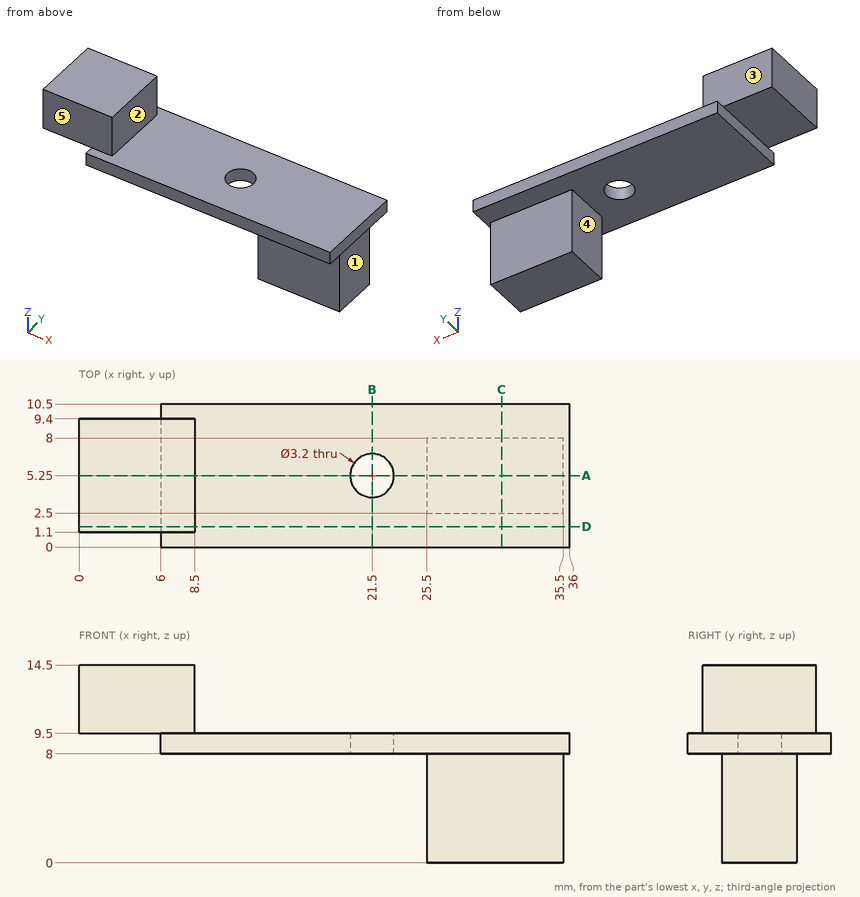
Answer from the drawing. Dimensions are ordinates in mm from the lowest x, y and z of the part. A direction names the side the tool comes from. Round coordinates to 2 decimals unless told otherwise and drop trailing zeros. Write each loop counter-clockwise with the first axis right and the second up, starting at its lowest first coordinate (ties: lowest second). Pieces come first, ordered by that corner, then holes. Notation, with made-up numbers: (5, 69.25) -> (48, 69.25) arc R14 cw to (48, 73.25) -> close; hole circle Ø4 at (-26.5, -3). An arc over 180 degrees is marked (long way). Answer in a Markdown table with one row per item. Add a question column.
1) Find section C-C, the plane x = 31. Determine the outline of the cut face in (y, z), and give its area (4 significant figures).
2) Find section B-B, the plane x = 21.5. Determine the outline of the cut face in (y, z), and give its area (4 significant figures).
3) Consider line 1 (Y direction, x = 21.5, z = 9.15); line 2 (Z direction, x = 3.5, y = 5.5); line 3 (X direction, y = 6.25, z = 10.5). Determine where each line is inside the solid, lowest interval first.
4) Find section A-A, the plane y = 5.25. Determine the outline of the cut face in (x, z), and give its area (3 significant figures).
5) Given P1, Ø5, axis at x = 28, y = 2.5, coming from the +Z side; P2, Ø3.5, axis at x = 21.5, y = 5.25, coming from the -Z side; P3, Ø4.5, axis at y = 5.5, z = 3.5, coming from the +X side; P4, Ø1.6, axis at y = 5, z = 9, coming from the -X side, each flat-ended and moving along its own axis, determine where each tip first touches the part or whether it passes through.
6) Find section D-D, the plane y = 1.5. Determine the outline of the cut face in (x, z).
7) Which of the six approach directions +Z, -Z, +X, -X, +Y, -Y give full straight-line access (tool end or side, diameter ignored) to the marked faces 1, 2, 3, 4 and 5?
Findings below:
| question | item | result |
|---|---|---|
| 1 | outline | (0, 8) -> (2.5, 8) -> (2.5, 0) -> (8, 0) -> (8, 8) -> (10.5, 8) -> (10.5, 9.5) -> (0, 9.5) -> close |
| 1 | area | 59.75 mm² |
| 2 | outline | (0, 8) -> (3.65, 8) -> (3.65, 9.5) -> (0, 9.5) -> close; (6.85, 8) -> (10.5, 8) -> (10.5, 9.5) -> (6.85, 9.5) -> close |
| 2 | area | 10.95 mm² |
| 3 | line 1 | 0 to 3.65, 6.85 to 10.5 |
| 3 | line 2 | 9.5 to 14.5 |
| 3 | line 3 | 0 to 8.5 |
| 4 | outline | (0, 9.5) -> (6, 9.5) -> (6, 8) -> (19.9, 8) -> (19.9, 9.5) -> (8.5, 9.5) -> (8.5, 14.5) -> (0, 14.5) -> close; (23.1, 8) -> (25.5, 8) -> (25.5, 0) -> (35.5, 0) -> (35.5, 8) -> (36, 8) -> (36, 9.5) -> (23.1, 9.5) -> close |
| 4 | area | 163 mm² |
| 5 | P1 | z = 9.5 |
| 5 | P2 | z = 8 |
| 5 | P3 | x = 35.5 |
| 5 | P4 | x = 0 |
| 6 | outline | (0, 9.5) -> (6, 9.5) -> (6, 8) -> (36, 8) -> (36, 9.5) -> (8.5, 9.5) -> (8.5, 14.5) -> (0, 14.5) -> close |
| 7 | face 1 | -Z, +X, +Y, -Y |
| 7 | face 2 | +Z, +X, +Y, -Y |
| 7 | face 3 | +Z, +X, -X, +Y |
| 7 | face 4 | -Z, -X, +Y, -Y |
| 7 | face 5 | +Z, +X, -X, -Y |
